Source: three-view drawing plus pictorial views. Frame: mm from the lowest corner of the part. A direction names the side the tool comes from. Coordinates: 2 decimals unless noted, no trailing zeros. Loops run counter-clockwise (first coordinate to the right, second up) from the corner with the lowest first, then second, coordinate; pieces in that order, holes last. Notation, with made-up numbers: M 77.25,-22 L 86.25,-22 A18 ccw 86.25,-12 Z; hole C 22.5,-16 d3. An arc over 180 degrees is marked long. Use a Markdown table: item, result. Add a question column.
1. Pin query (flat end, axial travel): pin 1 (4 mm diameter, centred on y = 9.5, z = 26.5, fed in from -X); pin 2 (1.5 mm diameter, centred on y = 10.5, z = 25.5, fed in from +X) (1 decimal); pin 3 (5 mm diameter, centred on y = 2, z = 19, fed in from +X). Return the tip coordinate at first contact, or that it passes through.
2. Section A-A on z = 23. Output: boundary loops of the cut face in (x, y) (1 decimal).
3. Line query: L1, parallel to X at y = 6.5, z = 11 (1 decimal); L2, parallel to X at y = 9, z = 5 (1 decimal). Output: solid intervals per line, ascending. Write a range as [from, to].
4. Draft query along X for the marked faces 1 and 2. Return one class per face: +X half, -X half, draft (parallel to the pull), parting line (faces both ways), or undercut.
5. Set-up query: the marked faces 3 and 4. Return all of +Z, -Z, +X, -X, +Y, -Y with unobstructed straight access to the full face (end or side cutting, diameter ignored); none if empty.
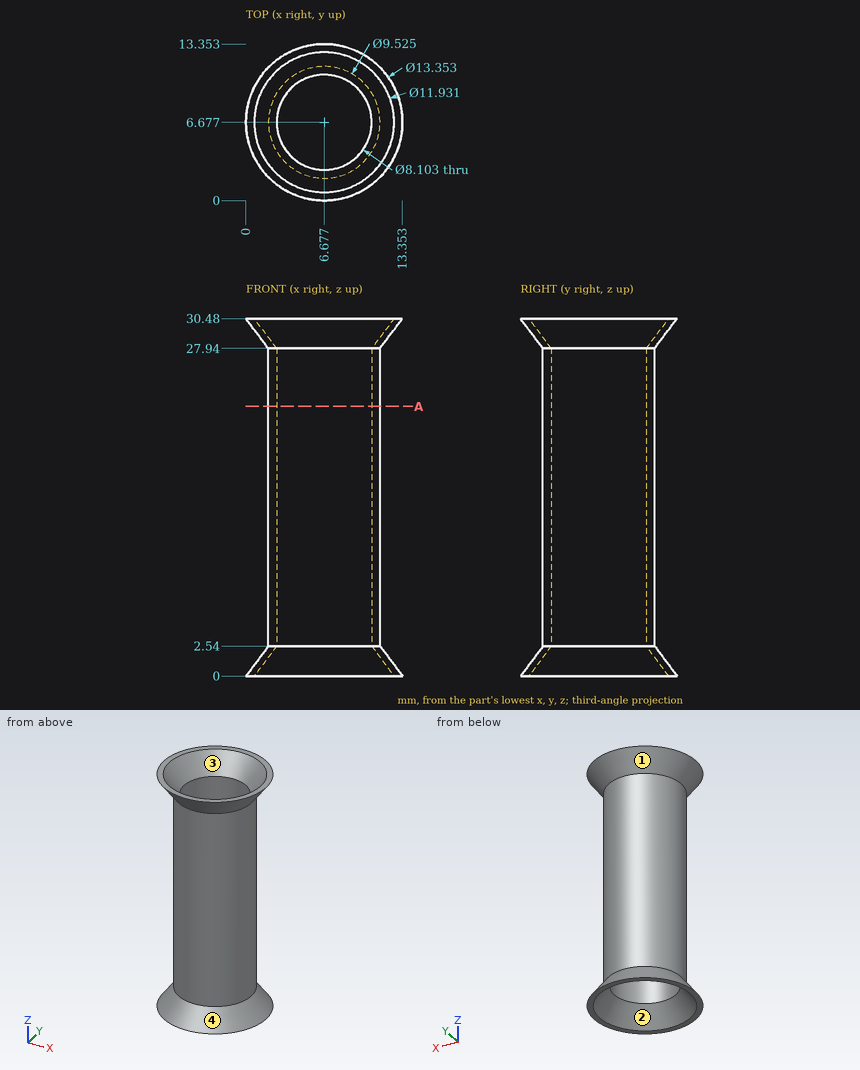
Answers below:
| question | item | result |
|---|---|---|
| 1 | pin 1 | stops at x = 1.99 |
| 1 | pin 2 | stops at x = 10.3 |
| 1 | pin 3 | stops at x = 10.91 |
| 2 | outline | C 6.7,6.7 d9.5; hole C 6.7,6.7 d8.1 |
| 3 | L1 | x = [1.9, 2.6], [10.7, 11.4] |
| 3 | L2 | x = [2.5, 3.4], [10, 10.8] |
| 4 | face 1 | parting line |
| 4 | face 2 | undercut |
| 5 | face 3 | +Z |
| 5 | face 4 | none |
